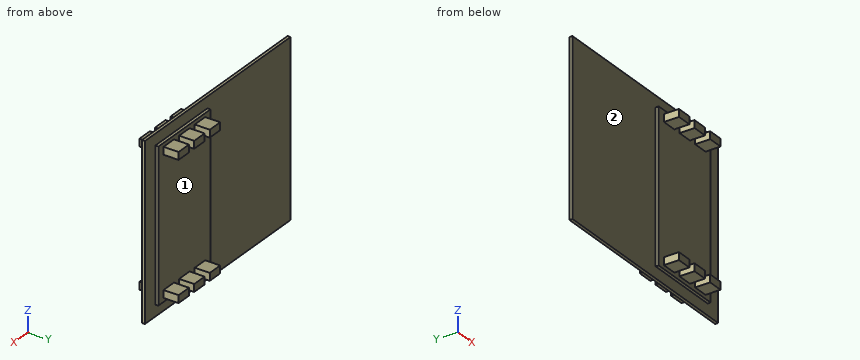
```python
from build123d import *

# Parameters (mm, degrees)
SKETCH1_W                = 177.8
SKETCH1_H                = 146.05
BOSS_EXTRUDE1_DEPTH      = 2.54
SKETCH2_W                = 63.5
SKETCH2_H                = 127
BOSS_EXTRUDE2_DEPTH      = 2.54
BOSS_EXTRUDE2_DEPTH_BACK = 5.08
SKETCH3_W                = 12.7
SKETCH3_H                = 6.35
BOSS_EXTRUDE3_DEPTH      = 12.7
BOSS_EXTRUDE3_DEPTH_BACK = 20.32


with BuildPart() as part:
    # Sketch1 → Boss-Extrude1 (new body)
    with BuildSketch(Plane(origin=(0, 0, 0), x_dir=(1, 0, 0), z_dir=(0, 1, 0))):
        Rectangle(SKETCH1_W, SKETCH1_H)
    extrude(amount=BOSS_EXTRUDE1_DEPTH)

    # Sketch2 → Boss-Extrude2 (add, two sides)
    with BuildSketch(Plane(origin=(0, 2.54, 0), x_dir=(1, 0, 0), z_dir=(0, 1, 0))) as boss_extrude2_sk:
        with Locations((44.45, 0)):
            Rectangle(SKETCH2_W, SKETCH2_H)
    extrude(amount=BOSS_EXTRUDE2_DEPTH)
    extrude(boss_extrude2_sk.sketch, amount=-BOSS_EXTRUDE2_DEPTH_BACK)

    # Sketch3 → Boss-Extrude3 (add, two sides)
    with BuildSketch(Plane(origin=(0, 5.08, 0), x_dir=(1, 0, 0), z_dir=(0, 1, 0))) as boss_extrude3_sk:
        with Locations((25.4, 57.15)):
            Rectangle(SKETCH3_W, SKETCH3_H)
        with Locations((44.45, 57.15)):
            Rectangle(SKETCH3_W, SKETCH3_H)
        with Locations((63.5, 57.15)):
            Rectangle(SKETCH3_W, SKETCH3_H)
        with Locations((63.5, -57.15)):
            Rectangle(SKETCH3_W, SKETCH3_H)
        with Locations((44.45, -57.15)):
            Rectangle(SKETCH3_W, SKETCH3_H)
        with Locations((25.4, -57.15)):
            Rectangle(SKETCH3_W, SKETCH3_H)
    extrude(amount=BOSS_EXTRUDE3_DEPTH)
    extrude(boss_extrude3_sk.sketch, amount=-BOSS_EXTRUDE3_DEPTH_BACK)


solid = part.part
```
Verification items for the finished model (mm, model axes). Face numbers are marked on the shaded views. Round coordinates to 2 decimals unless told otherwise and drop trailing zeros. Write each loop counter-clockwise with the first axis right and the second up, starting at its lowest first coordinate (ties: lowest second). Pieces come first, ordered by that corner, then holes. Notation, with made-up numbers: (71, -27.75) - (119, -27.75) arc R19 cw to (119, 5.25) - close; hole circle Ø4 at (2, -30). An arc over 180 degrees is marked (long way). Answer as a JSON object with one key per item and string values. Group by question number.
Q1. Section check C-C, the plane z = 47. Enter the section's corners in (x, y).
Q2. Go/stop test with flat-tipped pins: pin 1 Ø7 at (y, z) = (-11.5, -57.5) entering from +X; pin 2 Ø7 at (y, z) = (-10, 56) entering from -X; pin 3 Ø3 at (x, z) = (19.5, -12.5) entering from +Y; pin 4 Ø8 at (x, y) = (-66.5, -6) entering from -Z. Record where each tip stops, or that it passes through.
Q3. Thickness scan on line 1 (X direction, y = 15.5, z = 55.5); line 2 (Z direction, x = 27.5, y = -4) (3 decimals); line 3 (Y direction, x = -17, z = 46.5). Record the ranges inside material, lowest first.
Q4. Section check D-D, the plane x = -76. Enter the section's corners in (y, z) (3 decimals), plus the area to 3 significant figures.
Q5. Section check B-B, the plane x = 27. Enter the section's corners in (y, z) (3 decimals), plus the area to 3 significant figures.
Q6. Mould release check, pull along Z, two halves, no side actions. Record for the marked faces 1 and 2: released by +Z, released by -Z, zero draft, split by the parting line, or undercut.
Q7. Section check A-A, the plane y = 8.5. Enter the section's corners in (x, z) (3 decimals), plus the area to 3 significant figures.
Found:
{
 "1": {"outline": "(-88.9, 0) - (12.7, 0) - (12.7, -2.54) - (76.2, -2.54) - (76.2, 0) - (88.9, 0) - (88.9, 2.54) - (76.2, 2.54) - (76.2, 5.08) - (12.7, 5.08) - (12.7, 2.54) - (-88.9, 2.54) - close"},
 "2": {"pin 1": "stops at x = 69.85", "pin 2": "stops at x = 19.05", "pin 3": "stops at y = 5.08", "pin 4": "passes through"},
 "3": {"line 1": "x = 19.05 to 31.75, 38.1 to 50.8, 57.15 to 69.85", "line 2": "z = -60.325 to -53.975, 53.975 to 60.325", "line 3": "y = 0 to 2.54"},
 "4": {"outline": "(0, -73.025) - (2.54, -73.025) - (2.54, 73.025) - (0, 73.025) - close", "area": "371 mm^2"},
 "5": {"outline": "(-15.24, -60.325) - (-2.54, -60.325) - (-2.54, -63.5) - (0, -63.5) - (0, -73.025) - (2.54, -73.025) - (2.54, -63.5) - (5.08, -63.5) - (5.08, -60.325) - (17.78, -60.325) - (17.78, -53.975) - (5.08, -53.975) - (5.08, 53.975) - (17.78, 53.975) - (17.78, 60.325) - (5.08, 60.325) - (5.08, 63.5) - (2.54, 63.5) - (2.54, 73.025) - (0, 73.025) - (0, 63.5) - (-2.54, 63.5) - (-2.54, 60.325) - (-15.24, 60.325) - (-15.24, 53.975) - (-2.54, 53.975) - (-2.54, -53.975) - (-15.24, -53.975) - close", "area": "1,340 mm^2"},
 "6": {"face 1": "undercut", "face 2": "zero draft"},
 "7": {"outline": "(19.05, -60.325) - (31.75, -60.325) - (31.75, -53.975) - (19.05, -53.975) - close; (19.05, 53.975) - (31.75, 53.975) - (31.75, 60.325) - (19.05, 60.325) - close; (38.1, -60.325) - (50.8, -60.325) - (50.8, -53.975) - (38.1, -53.975) - close; (38.1, 53.975) - (50.8, 53.975) - (50.8, 60.325) - (38.1, 60.325) - close; (57.15, -60.325) - (69.85, -60.325) - (69.85, -53.975) - (57.15, -53.975) - close; (57.15, 53.975) - (69.85, 53.975) - (69.85, 60.325) - (57.15, 60.325) - close", "area": "484 mm^2"}
}
